```python
from build123d import *

# Parameters (mm, degrees)
SKETCH1_W           = 155
SKETCH1_H           = 110
BOSS_EXTRUDE1_DEPTH = 2
SKETCH2_W           = 151
SKETCH2_H           = 106
BOSS_EXTRUDE2_DEPTH = 1.5
SKETCH3_W           = 15
SKETCH3_H           = 15
CUT_EXTRUDE2_DEPTH  = 3.5
SKETCH5_W           = 4
SKETCH5_H           = 100
CUT_EXTRUDE3_DEPTH  = 3.5


with BuildPart() as part:
    # Sketch1 → Boss-Extrude1 (new body)
    with BuildSketch(Plane.XY):
        with Locations((77.5, 55)):
            Rectangle(SKETCH1_W, SKETCH1_H)
    extrude(amount=BOSS_EXTRUDE1_DEPTH)

    # Sketch2 → Boss-Extrude2 (add)
    with BuildSketch(Plane.XY.offset(2)):
        with Locations((77.5, 55)):
            Rectangle(SKETCH2_W, SKETCH2_H)
    extrude(amount=BOSS_EXTRUDE2_DEPTH)

    # Sketch3 → Cut-Extrude2 (cut)
    with BuildSketch(Plane.XY.offset(3.5)):
        with Locations((145.5, 55)):
            Rectangle(SKETCH3_W, SKETCH3_H)
    extrude(amount=-CUT_EXTRUDE2_DEPTH, mode=Mode.SUBTRACT)

    # Sketch5 → Cut-Extrude3 (cut)
    with BuildSketch(Plane.XY.offset(3.5)):
        with Locations((17, 55)):
            Rectangle(SKETCH5_W, SKETCH5_H)
        with Locations((7, 55)):
            Rectangle(SKETCH5_W, SKETCH5_H)
        with Locations((27, 55)):
            Rectangle(SKETCH5_W, SKETCH5_H)
        with Locations((37, 55)):
            Rectangle(SKETCH5_W, SKETCH5_H)
        with Locations((47, 55)):
            Rectangle(SKETCH5_W, SKETCH5_H)
        with Locations((57, 55)):
            Rectangle(SKETCH5_W, SKETCH5_H)
        with Locations((67, 55)):
            Rectangle(SKETCH5_W, SKETCH5_H)
        with Locations((77, 55)):
            Rectangle(SKETCH5_W, SKETCH5_H)
        with Locations((87, 55)):
            Rectangle(SKETCH5_W, SKETCH5_H)
        with Locations((97, 55)):
            Rectangle(SKETCH5_W, SKETCH5_H)
        with Locations((107, 55)):
            Rectangle(SKETCH5_W, SKETCH5_H)
        with Locations((117, 55)):
            Rectangle(SKETCH5_W, SKETCH5_H)
        with Locations((127, 55)):
            Rectangle(SKETCH5_W, SKETCH5_H)
    extrude(amount=-CUT_EXTRUDE3_DEPTH, mode=Mode.SUBTRACT)


solid = part.part
```
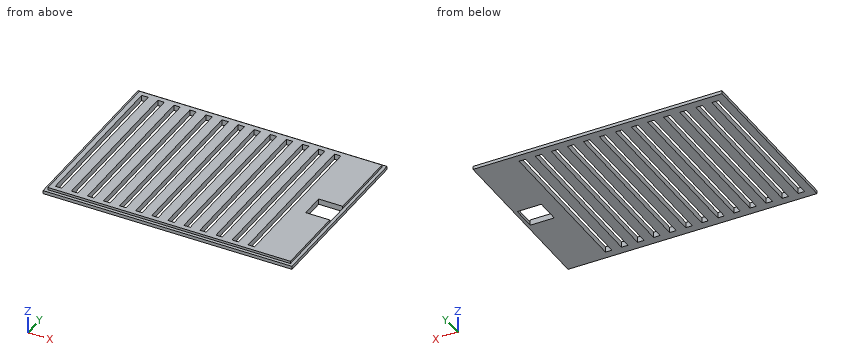
The model under review builds one solid part; all positions refer to its coordinate system, in mm. Round coordinates to 2 decimals unless told otherwise and drop trailing zeros. Order: outer loops, then holes, each group sorted by start corner. A loop starts at its lowest first (then second) coordinate and runs counter-clockwise, first axis right, second up. Notation, with made-up numbers: (3.25, -21.5) -> (35.25, -21.5) arc R35 cw to (35.25, 12.5) -> close; hole circle Ø9 at (28, 49). An arc over 180 degrees is marked (long way). Use a Markdown table: item, result.
Q1. We need section A-A on y = 16.5. State how many separate pieces and enclosed holes the cut face has, then the cut area to 4 significant figures.
Values:
| item | result |
|---|---|
| separate pieces | 14 |
| enclosed holes | 0 |
| area | 354.5 mm^2 |
Q2. We need section C-C on x = 52. Write out the cut boundary in (y, z), then the cut area to 3 significant figures.
Values:
| item | result |
|---|---|
| outline | (0, 0) -> (110, 0) -> (110, 2) -> (108, 2) -> (108, 3.5) -> (2, 3.5) -> (2, 2) -> (0, 2) -> close |
| area | 379 mm^2 |
Q3. Clearance check with a flat-ended pin moving along its axis: P1, Ø1.6, axis at x = 104, z = 3, coming from the -Y side. State where the tip first meets the part, or that it passes through.
Values:
| item | result |
|---|---|
| P1 | stops at y = 2 |
Q4. For line 1 (Y direction, x = 143.5, z = 0.75); line 2 (Y direction, x = 105.5, z = 1.55); line 3 (Y direction, x = 12, z = 2.1), list the stretches that pass through material, from the lowest coordinate up.
Values:
| item | result |
|---|---|
| line 1 | y = 0 to 47.5, 62.5 to 110 |
| line 2 | y = 0 to 5, 105 to 110 |
| line 3 | y = 2 to 108 |
